Part model, mm, in its own coordinate system. A direction names the side the tool comes from. Give positions to 0.01 mm unless a question says otherwise; leave off trailing zeros. Write each loop counter-clockwise with the first axis right and the second up, starting at its lowest first coordinate (ties: lowest second). Pieces come first, ordered by that corner, then holes. Notation, with made-up numbers: (52.5, 55) - (88.5, 55) arc R12 cw to (88.5, 77) - close; hole circle Ø6 at (-32, 58.25). An arc over 180 degrees is marked (long way). Answer as a JSON object with one key per item and string values. Group by question number.
```python
from build123d import *

# Parameters (mm, degrees)
SKETCH1_W            = 185
SKETCH1_H            = 142
BOSS_EXTRUDE1_DEPTH  = 23
SKETCH12_W           = 80
SKETCH12_H           = 100
BOSS_EXTRUDE6_DEPTH  = 53
SHELL1_T             = -5
SKETCH11_R           = 6.25
CUT_EXTRUDE2_DEPTH   = 6
FILLET1_R            = 2
SKETCH13_R           = 1.95
CUT_EXTRUDE3_DEPTH   = 54
SKETCH15_W           = 10
SKETCH15_H           = 5
BOSS_EXTRUDE8_DEPTH  = 10
SKETCH16_W           = 10
SKETCH16_H           = 5
BOSS_EXTRUDE9_DEPTH  = 10
SKETCH17_W           = 10
SKETCH17_H           = 5
BOSS_EXTRUDE10_DEPTH = 10
FILLET2_R            = 2
SKETCH18_R           = 1.5
CUT_EXTRUDE4_DEPTH   = 10
SKETCH19_R           = 7.5
BOSS_EXTRUDE11_DEPTH = 18
FILLET3_R            = 2


with BuildPart() as part:
    # Sketch1 → Boss-Extrude1 (new body)
    with BuildSketch(Plane(origin=(0, 0, 0), x_dir=(1, 0, 0), z_dir=(0, 1, 0))):
        with Locations((92.5, 71)):
            Rectangle(SKETCH1_W, SKETCH1_H)
    extrude(amount=BOSS_EXTRUDE1_DEPTH)

    # Sketch12 → Boss-Extrude6 (add)
    with BuildSketch(Plane(origin=(0, 0, 0), x_dir=(1, 0, 0), z_dir=(0, 1, 0))):
        with Locations((40, 140)):
            Rectangle(SKETCH12_W, SKETCH12_H)
    extrude(amount=BOSS_EXTRUDE6_DEPTH)

    # Shell1
    shell1_openings = [part.faces().sort_by_distance(p)[0] for p in [
        (88.333333333, 0, -110.666666667),
        (185, 11.5, -71),
        (0, 25.333333333, -93.333333333),
    ]]
    offset(amount=SHELL1_T, openings=shell1_openings, kind=Kind.INTERSECTION)

    # Sketch11 → Cut-Extrude2 (cut)
    with BuildSketch(Plane.XY):
        with Locations((18.4375, 9.5)):
            Circle(SKETCH11_R)
        with Locations((43.088852194, 9.5)):
            Circle(SKETCH11_R)
        with Locations((67.740204388, 9.5)):
            Circle(SKETCH11_R)
        with Locations((92.391556582, 9.5)):
            Circle(SKETCH11_R)
        with Locations((117.042908776, 9.5)):
            Circle(SKETCH11_R)
        with Locations((141.69426097, 9.5)):
            Circle(SKETCH11_R)
        with Locations((166.345613164, 9.5)):
            Circle(SKETCH11_R)
    extrude(amount=-CUT_EXTRUDE2_DEPTH, mode=Mode.SUBTRACT)

    # Fillet1
    fillet1_edges = [part.edges().sort_by_distance(p)[0] for p in [
        (92.5, 18, -5),
        (130, 18, -137),
        (37.5, 48, -95),
        (75, 48, -140),
        (37.5, 48, -185),
    ]]
    fillet(fillet1_edges, radius=FILLET1_R)

    # Sketch13 → Cut-Extrude3 (cut, through all)
    with BuildSketch(Plane(origin=(0, 53, 0), x_dir=(1, 0, 0), z_dir=(0, 1, 0))):
        with Locations((15, 100.5)):
            Circle(SKETCH13_R)
        with Locations((15, 179.5)):
            Circle(SKETCH13_R)
        with Locations((65, 179.5)):
            Circle(SKETCH13_R)
        with Locations((65, 100.5)):
            Circle(SKETCH13_R)
    extrude(amount=-CUT_EXTRUDE3_DEPTH, mode=Mode.SUBTRACT)

    # Sketch15 → Boss-Extrude8 (add)
    with BuildSketch(Plane.XY):
        with Locations((5, 2.5)):
            Rectangle(SKETCH15_W, SKETCH15_H)
        with Locations((180, 2.5)):
            Rectangle(SKETCH15_W, SKETCH15_H)
    extrude(amount=BOSS_EXTRUDE8_DEPTH)

    # Sketch16 → Boss-Extrude9 (add)
    with BuildSketch(Plane(origin=(0, 0, -190), x_dir=(-1, 0, 0), z_dir=(0, 0, -1))):
        with Locations((-5, 2.5)):
            Rectangle(SKETCH16_W, SKETCH16_H)
        with Locations((-75, 2.5)):
            Rectangle(SKETCH16_W, SKETCH16_H)
    extrude(amount=BOSS_EXTRUDE9_DEPTH)

    # Sketch17 → Boss-Extrude10 (add)
    with BuildSketch(Plane(origin=(0, 0, -142), x_dir=(-1, 0, 0), z_dir=(0, 0, -1))):
        with Locations((-180, 2.5)):
            Rectangle(SKETCH17_W, SKETCH17_H)
        with Locations((-85, 2.5)):
            Rectangle(SKETCH17_W, SKETCH17_H)
    extrude(amount=BOSS_EXTRUDE10_DEPTH)

    # Fillet2
    fillet2_edges = [part.edges().sort_by_distance(p)[0] for p in [
        (175, 2.5, -142),
        (180, 5, -142),
        (90, 2.5, -142),
        (85, 5, -142),
        (80, 5, -147),
        (80, 2.5, -152),
        (75, 5, -190),
        (70, 2.5, -190),
        (180, 5, 0),
        (5, 5, 0),
        (10, 2.5, -190),
        (5, 5, -190),
    ]]
    fillet(fillet2_edges, radius=FILLET2_R)

    # Sketch18 → Cut-Extrude4 (cut)
    with BuildSketch(Plane(origin=(0, 5, 0), x_dir=(1, 0, 0), z_dir=(0, 1, 0))):
        with Locations((180, 147)):
            Circle(SKETCH18_R)
        with Locations((85, 147)):
            Circle(SKETCH18_R)
        with Locations((5, -5)):
            Circle(SKETCH18_R)
        with Locations((180, -5)):
            Circle(SKETCH18_R)
        with Locations((75, 195)):
            Circle(SKETCH18_R)
        with Locations((5, 195)):
            Circle(SKETCH18_R)
    extrude(amount=-CUT_EXTRUDE4_DEPTH, mode=Mode.SUBTRACT)

    # Sketch19 → Boss-Extrude11 (add)
    with BuildSketch(Plane(origin=(0, 18, 0), x_dir=(-1, 0, 0), z_dir=(0, -1, 0))):
        with Locations((-165, 71)):
            Circle(SKETCH19_R)
        with Locations((-92.5, 71)):
            Circle(SKETCH19_R)
        with Locations((-20, 71)):
            Circle(SKETCH19_R)
    extrude(amount=BOSS_EXTRUDE11_DEPTH)

    # Fillet3
    fillet3_edges = [part.edges().sort_by_distance(p)[0] for p in [
        (172.5, 18, -71),
        (100, 18, -71),
        (27.5, 18, -71),
    ]]
    fillet(fillet3_edges, radius=FILLET3_R)


solid = part.part
```
1) Band-saw the part on B-B (z = -71). List the corners of the cut face in (x, y).
2) Band-saw the part on C-C (y = 42). List the corners of the cut face in (x, z).
3) Probe line 1 (Z direction, x = 108.5, y = 2); line 2 (X direction, y = 2, z = 5); line 3 (Z direction, x = 21, y = 43). List the from-to ranges inside material, lowest first.
4) Which spindle directions (+Z, -Z, +X, -X, +Y, -Y) get a long thin tool onto all of the face, cutting with end or side? Do faces 4 (the flat face through (129, 8, -137)), 5 (the flat face through (5, 5, 7)), 6 (the flat face through (75, 28, -149)). Say none if no direction does.
5) Band-saw the part on D-D (x = 165). List the corners of the cut face in (y, z).
6) Band-saw the part on A-A (x = 20). List the corners of the cut face in (y, z), plus the area to 3 significant figures.
7) Mould opens along X. For faces 1 (the cylindrical face through (87.43, 5.7, -2.46)), 2 (the flat face through (185, 18.3, -64.6)), 3 (the flat face through (180, 5, -149)) say: pulls with the +X half, pulls with the -X half, needs draft (parallel to the pull), parting line crosses it, or undercut.
8) Drop flat-ended pins along their axis: P1, Ø9, axis at x = 59.5, y = 39, coming from the +Z side; P2, Ø14, axis at x = 31.5, y = 27.5, coming from the +Z side; P3, Ø4, axis at y = 3, z = -197.5, coming from the +X side; P4, Ø3, axis at x = 65, z = -100.5, coming from the +Y side. Give the stop position or say it passes through.
Verdict:
{
 "1": {"outline": "(0, 18) - (10.5, 18) arc R2 cw to (12.5, 16) - (12.5, 0) - (27.5, 0) - (27.5, 16) arc R2 cw to (29.5, 18) - (83, 18) arc R2 cw to (85, 16) - (85, 0) - (100, 0) - (100, 16) arc R2 cw to (102, 18) - (155.5, 18) arc R2 cw to (157.5, 16) - (157.5, 0) - (172.5, 0) - (172.5, 16) arc R2 cw to (174.5, 18) - (185, 18) - (185, 23) - (0, 23) - close"},
 "2": {"outline": "(0, -190) - (80, -190) - (80, -90) - (0, -90) - (0, -95) - (75, -95) - (75, -185) - (0, -185) - close"},
 "3": {"line 1": "-142 to -137, -5 to 0", "line 2": "0 to 3.5, 6.5 to 10, 175 to 178.5, 181.5 to 185", "line 3": "-190 to -185, -95 to -90"},
 "4": {"face 4": "+X, -X, -Y", "face 5": "+Z, +X, -X, +Y", "face 6": "-X, -Y"},
 "5": {"outline": "(0, -142) - (23, -142) - (23, 0) - (15.6, 0) - (15.6, -5) - (16, -5) arc R2 cw to (18, -7) - (18, -61.5) arc R2 cw to (16, -63.5) - (0, -63.5) - (0, -78.5) - (16, -78.5) arc R2 cw to (18, -80.5) - (18, -135) arc R2 cw to (16, -137) - (0, -137) - close; (0, -5) - (3.4, -5) - (3.4, 0) - (0, 0) - close"},
 "6": {"outline": "(0, -190) - (53, -190) - (53, -90) - (23, -90) - (23, 0) - (15.55, 0) - (15.55, -5) - (16, -5) arc R2 cw to (18, -7) - (18, -61.5) arc R2 cw to (16, -63.5) - (0, -63.5) - (0, -78.5) - (16, -78.5) arc R2 cw to (18, -80.5) - (18, -95) - (46, -95) arc R2 cw to (48, -97) - (48, -183) arc R2 cw to (46, -185) - (0, -185) - close; (0, -5) - (3.45, -5) - (3.45, 0) - (0, 0) - close", "area": "1,640 mm2"},
 "7": {"face 1": "undercut", "face 2": "pulls with the +X half", "face 3": "needs draft"},
 "8": {"P1": "z = -90", "P2": "z = 0", "P3": "x = 80", "P4": "through"}
}
